Geometry: see drawing. Coordinates: mm, zero at the bounding-box minimum. A direction names the side the tool comes from. Coordinates: 2 decimals unless noted, no trailing zeros. Order: outer loops, then holes, each group sorted by start corner. A loop starts at its lowest first (then second) coordinate and runs counter-clockwise, first axis right, second up. Notation, with made-up numbers: (-20, -15) - (-16, -15) arc R16 ccw to (-16, -10) - close; hole circle Ø7 at (0, -12.5). An arc over 180 degrees is marked (long way). Use a Markdown table: item, result. Add a question column.
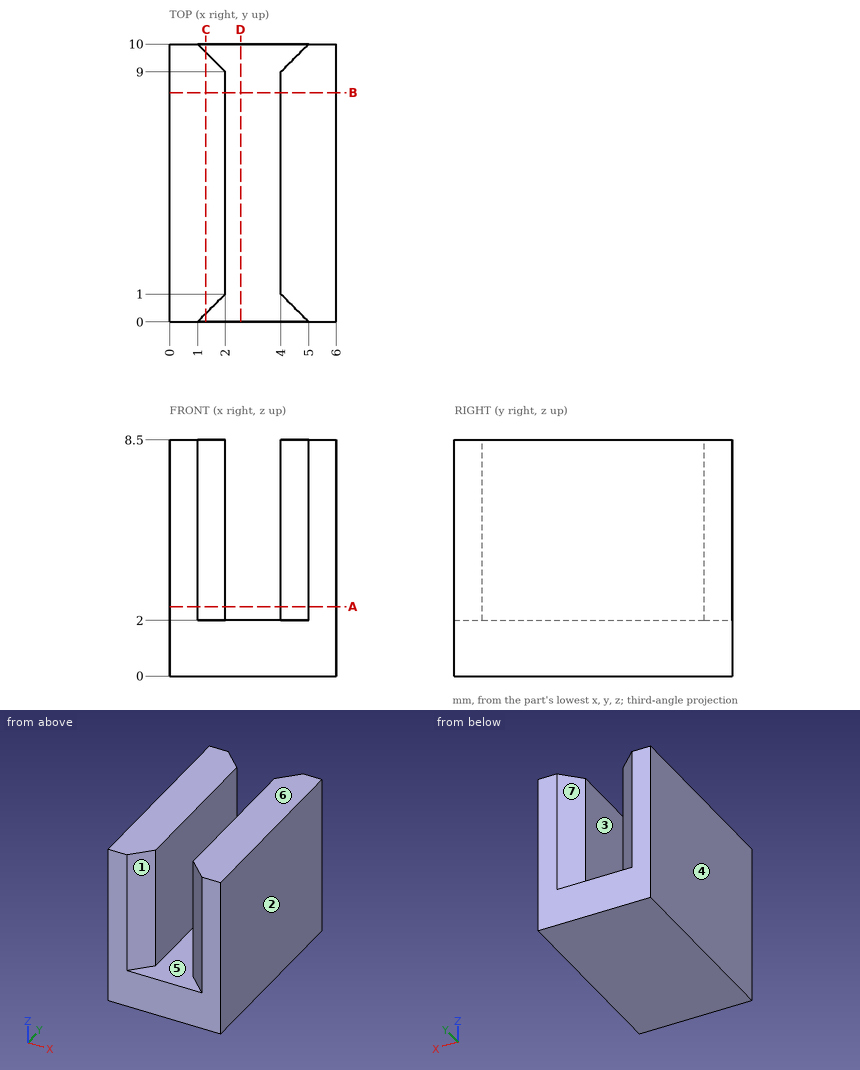
1) Draft query along X for the marked faces 4, 5, 6 and 7. Return one class per face: released by +X, released by -X, zero draft, split by the parting line, or undercut.
2) Section query D-D (x = 2.55). Return the cut outline in (y, z), and give its area (3 significant figures).
3) Section query B-B (y = 8.25). Return the cut outline in (x, z), and give its area (3 significant figures).
4) Line query: line 1 (X direction, y = 1.25, z = 8.25); line 2 (Z direction, x = 3.6, y = 2); line 3 (X direction, y = 0.5, z = 3). Output: solid intervals per line, ascending. Write a range as from..to.
5) Access query for the marked faces 1, 2 and 3. Directions: +Z, -Z, +X, -X, +Y, -Y. A direction counts if a zero-diameter tool reaches every point of the face in a straight line with its end or side. Return the directions, or none.
6) First-contact query: pin 1 (1 mm diameter, centred on x = 3, y = 8.5, fed in from +Z); pin 2 (3 mm diameter, centred on y = 4.5, z = 6.5, fed in from -X). Flat tips, straight axial feed; report the tip coordinate or a pass-through.
7) Section query C-C (x = 1.3). Return the cut outline in (y, z).
8) Section query A-A (z = 2.5). Return the cut outline in (x, y).
From the geometry:
| question | item | result |
|---|---|---|
| 1 | face 4 | released by -X |
| 1 | face 5 | undercut |
| 1 | face 6 | zero draft |
| 1 | face 7 | undercut |
| 2 | outline | (0, 0) - (10, 0) - (10, 2) - (0, 2) - close |
| 2 | area | 20.0 mm^2 |
| 3 | outline | (0, 0) - (6, 0) - (6, 8.5) - (4, 8.5) - (4, 2) - (2, 2) - (2, 8.5) - (0, 8.5) - close |
| 3 | area | 38.0 mm^2 |
| 4 | line 1 | x = 0..2, 4..6 |
| 4 | line 2 | z = 0..2 |
| 4 | line 3 | x = 0..1.5, 4.5..6 |
| 5 | face 1 | +Z, -Y |
| 5 | face 2 | +Z, -Z, +X, +Y, -Y |
| 5 | face 3 | +Z, +Y, -Y |
| 6 | pin 1 | stops at z = 2 |
| 6 | pin 2 | stops at x = 0 |
| 7 | outline | (0, 0) - (10, 0) - (10, 2) - (9.7, 2) - (9.7, 8.5) - (0.3, 8.5) - (0.3, 2) - (0, 2) - close |
| 8 | outline | (0, 0) - (1, 0) - (2, 1) - (2, 9) - (1, 10) - (0, 10) - close; (4, 1) - (5, 0) - (6, 0) - (6, 10) - (5, 10) - (4, 9) - close |
